Autodesk Inventor part; units mm, degrees
ref_plane "YZ Plane" through (0, 0, 0) normal (1, 0, 0) x (0, 1, 0)
ref_plane "XZ Plane" through (0, 0, 0) normal (0, 1, 0) x (-1, 0, 0)
ref_plane "XY Plane" through (0, 0, 0) normal (0, 0, 1) x (1, 0, 0)
sketch "Sketch1" plane through (0, 0, 0) normal (1, 0, 0) x (0, 1, 0)
  point P0 (0, 0)
sketch "Sketch2" plane through (0, 0, 0) normal (1, 0, 0) x (0, 1, 0)
  line L0 (57.15, 57.15) -> (-57.15, 57.15)
  line L1 (-57.15, 57.15) -> (-57.15, -57.15)
  line L2 (-57.15, -57.15) -> (57.15, -57.15)
  line L3 (57.15, -57.15) -> (57.15, 57.15)
  line L4 (57.15, 57.15) -> (-57.15, -57.15) construction
  line L5 (-57.15, 57.15) -> (57.15, -57.15) construction
  point P0 (0, 0)
  dimension "d0" = 114.3
  dimension "d1" = 114.3
extrude "Extrusion1" add sketch "Sketch2" along normal blind 254
sketch "Sketch3" plane through (0, 57.15, 57.15) normal (0, 1, 0) x (1, 0, 0)
  line L0 (3.9878, 110.3122) -> (250.0122, 110.3122)
  line L1 (250.0122, 110.3122) -> (250.0122, 3.9878)
  line L2 (250.0122, 3.9878) -> (3.9878, 3.9878)
  line L3 (3.9878, 3.9878) -> (3.9878, 110.3122)
  line L4 (0, 114.3) -> (254, 114.3)
  line L5 (0, 114.3) -> (0, 0)
  line L6 (0, 0) -> (254, 0)
  line L7 (254, 114.3) -> (254, 0)
  point P0 (0, 57.15)
  dimension "d4" = 3.9878
  dimension "d5" = 3.9878
  dimension "d6" = 3.9878
  dimension "d7" = 3.9878
extrude "Extrusion2" cut sketch "Sketch3" against normal blind 110.3122 contours L0 L1 L2 L3
sketch "Sketch5" plane through (0, -57.15, 57.15) normal (0, 0, 1) x (1, 0, 0)
  circle A0 centre (57.15, 50.8) radius 5.0038
  circle A1 centre (196.85, 50.8) radius 5.0038
  line L0 (0, 0) -> (254, 0)
  line L1 (0, 114.3) -> (0, 0)
  line L2 (254, 114.3) -> (254, 0)
  point P0 (0, 57.15)
  dimension "d19" = 10.0076
  dimension "d20" = 10.0076
  dimension "d21" = 50.8
  dimension "d22" = 50.8
  dimension "d23" = 57.15
  dimension "d24" = 57.15
extrude "Extrusion3" cut sketch "Sketch5" against normal through all
sketch "Sketch6" plane through (0, -57.15, -57.15) normal (0, -1, 0) x (1, 0, 0)
  circle A0 centre (50.8, 57.15) radius 1.9939
  circle A1 centre (76.2, 57.15) radius 1.9939
  circle A2 centre (177.8, 57.15) radius 1.9939
  circle A3 centre (203.2, 57.15) radius 1.9939
  line L0 (0, 114.3) -> (254, 114.3)
  line L1 (0, 114.3) -> (0, 0)
  line L2 (254, 114.3) -> (254, 0)
  point P0 (0, 57.15)
  dimension "d27" = 3.9878
  dimension "d28" = 3.9878
  dimension "d29" = 3.9878
  dimension "d30" = 3.9878
  dimension "d31" = 57.15
  dimension "d32" = 57.15
  dimension "d33" = 57.15
  dimension "d34" = 57.15
  dimension "d35" = 50.8
  dimension "d36" = 50.8
  dimension "d37" = 76.2
  dimension "d38" = 76.2
extrude "Extrusion4" cut sketch "Sketch6" against normal through all
fillet "Fillet3" radius 1.999 4 edges at (250.0122, 57.15, 0) (127, 57.15, -53.1622) (127, 57.15, 53.1622) (3.9878, 57.15, 0)
sketch "Sketch7" plane through (0, 0, 0) normal (-1, 0, 0) x (0, 0, 1)
  circle A0 centre (-27.1526, 27.1526) radius 9.9949
  circle A1 centre (27.1526, 27.1526) radius 9.9949
  line L0 (-31.75, -11.7602) -> (31.75, -11.7602)
  line L1 (31.75, -11.7602) -> (31.75, -31.75)
  line L2 (31.75, -31.75) -> (-31.75, -31.75)
  line L3 (-31.75, -31.75) -> (-31.75, -11.7602)
  line L4 (57.15, -57.15) -> (-57.15, -57.15)
  line L5 (57.15, 57.15) -> (57.15, -57.15)
  line L6 (-57.15, 57.15) -> (57.15, 57.15)
  line L7 (-57.15, -57.15) -> (-57.15, 57.15)
  point P0 (0, 0)
  dimension "d43" = 19.9898
  dimension "d44" = 19.9898
  dimension "d45" = 63.5
  dimension "d46" = 19.9898
  dimension "d47" = 25.4
  dimension "d48" = 25.4
  dimension "d49" = 29.9974
  dimension "d50" = 29.9974
  dimension "d51" = 29.9974
  dimension "d52" = 29.9974
sketch "Sketch8" plane through (0, 0, 0) normal (-1, 0, 0) x (0, 0, 1)
  point P0 (0, 0)
extrude "Extrusion5" cut sketch "Sketch7" against normal blind 3.9878 contours A0 | A1 | L0 L1 L2 L3
sketch "Sketch9" plane through (254, 0, 0) normal (1, 0, 0) x (0, 0, -1)
  circle A0 centre (-38.1, 38.1) radius 1.9939
  circle A1 centre (38.1, 38.1) radius 1.9939
  circle A2 centre (-38.1, -38.1) radius 1.9939
  circle A3 centre (38.1, -38.1) radius 1.9939
  line L0 (57.15, 57.15) -> (-57.15, 57.15)
  line L1 (-57.15, 57.15) -> (-57.15, -57.15)
  line L2 (57.15, -57.15) -> (57.15, 57.15)
  line L3 (-57.15, -57.15) -> (57.15, -57.15)
  point P0 (0, 0)
  dimension "d55" = 3.9878
  dimension "d56" = 3.9878
  dimension "d57" = 3.9878
  dimension "d58" = 3.9878
  dimension "d59" = 19.05
  dimension "d60" = 19.05
  dimension "d61" = 19.05
  dimension "d62" = 19.05
  dimension "d63" = 19.05
  dimension "d64" = 19.05
  dimension "d65" = 19.05
  dimension "d66" = 19.05
sketch "Sketch10" plane through (254, 0, 0) normal (1, 0, 0) x (0, 0, -1)
  point P0 (0, 0)
extrude "Extrusion6" cut sketch "Sketch9" against normal blind 3.9878 contours A0 | A1 | A2 | A3
sketch "Sketch16" plane through (0, -57.15, 57.15) normal (0, 0, 1) x (1, 0, 0)
  point P0 (0, 57.15)
sketch "Sketch17" plane through (0, -57.15, 57.15) normal (0, 0, 1) x (1, 0, 0)
  point P0 (0, 57.15)
sketch "Sketch18" plane through (0, 0, 0) normal (-1, 0, 0) x (0, 0, 1)
  circle A0 centre (0, 31.75) radius 1.9939
  circle A1 centre (0, -44.45) radius 1.9939
  line L0 (-57.15, 57.15) -> (57.15, 57.15)
  line L1 (57.15, -57.15) -> (-57.15, -57.15)
  point P0 (0, 0)
  dimension "d89" = 3.9878
  dimension "d90" = 3.9878
  dimension "d91" = 25.4
  dimension "d92" = 12.7
extrude "Extrusion11" add sketch "Sketch18" along normal blind 25.4
sketch "Sketch19" plane through (0, 0, 0) normal (-1, 0, 0) x (0, 0, 1)
  point P0 (0, 0)
properties part number "pranshu part" material "PBT Plastic"
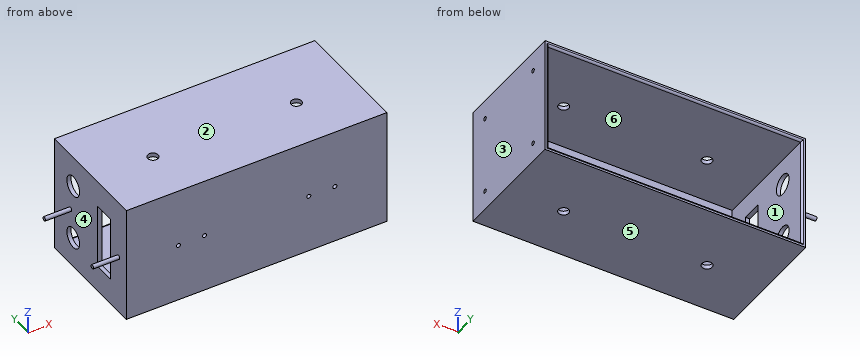
Verification items for the finished model (mm, model axes). Face numbers are marked on the shaded views. A direction names the side the tool comes from. Coordinates: 2 decimals unless noted, no trailing zeros. Write each loop counter-clockwise with the first axis right and the second up, starting at its lowest first coordinate (ties: lowest second). Pieces come first, ordered by that corner, then holes. Notation, with made-up numbers: M 19.25,2 L 49.25,2 A26 ccw 49.25,38 Z; hole C -19.75,41 d7. An arc over 180 degrees is marked long. Use a Markdown table: item, result.
Q1. Sectioned sample at B-B, the plane x = 57.15. Record the boundary of the cut face in (y, z).
Reply:
| item | result |
|---|---|
| outline | M -57.15,-57.15 L -11.35,-57.15 L -11.35,-53.16 L -53.16,-53.16 L -53.16,53.16 L -11.35,53.16 L -11.35,57.15 L -57.15,57.15 Z; M -1.35,-57.15 L 57.15,-57.15 L 57.15,-55.16 A2 ccw 55.15,-53.16 L -1.35,-53.16 Z; M -1.35,53.16 L 55.15,53.16 A2 ccw 57.15,55.16 L 57.15,57.15 L -1.35,57.15 Z |
Q2. Draft check along X on the marked faces 1, 2, 3 and 4. Enter one of: +X half, -X half, draft (parallel to the pull), parting line (faces both ways), or undercut.
Reply:
| item | result |
|---|---|
| face 1 | undercut |
| face 2 | draft |
| face 3 | +X half |
| face 4 | -X half |
Q3. Set-up check for the marked faces 5 and 6: record each of +Z, -Z, +X, -X, +Y, -Y from which the full face is reachable in a straight line by a thin tool's end or side.
Reply:
| item | result |
|---|---|
| face 5 | -Z, +X, -X, +Y, -Y |
| face 6 | +Y |
Q4. Sectioned sample at A-A, the plane y = 3. Record the boundary of the cut face in (x, z), plus the area to 3 significant figures.
Reply:
| item | result |
|---|---|
| outline | M 0,-57.15 L 254,-57.15 L 254,57.15 L 0,57.15 Z; hole M 3.99,-53.16 L 250.01,-53.16 L 250.01,53.16 L 3.99,53.16 Z |
| area | 2,870 mm² |
Q5. Sectioned sample at C-C, the plane z = -46.5. Record the boundary of the cut face in (x, y), plus the area to 3 significant figures.
Reply:
| item | result |
|---|---|
| outline | M 0,-57.15 L 254,-57.15 L 254,57.15 L 252.01,57.15 A2 ccw 250.01,55.15 L 250.01,-53.16 L 3.99,-53.16 L 3.99,55.15 A2 ccw 1.99,57.15 L 0,57.15 Z |
| area | 1,890 mm² |
Q6. Go/stop test with flat-tipped pins: P1, Ø1, axis at x = 209.5, z = -36.5, coming from the +Y side; P2, Ø10, axis at y = 22.5, z = 25, coming from the -X side; P3, Ø2.5, axis at y = 38.1, z = -38.1, coming from the +X side. Record where each tip stops, or that it passes through.
Reply:
| item | result |
|---|---|
| P1 | stops at y = -53.16 |
| P2 | stops at x = 0 |
| P3 | stops at x = 3.99 |
Q7. Thickness scan on line 1 (X direction, y = -6, z = 55); line 2 (X direction, y = -33.5, z = -27); line 3 (Z direction, x = 138, y = -8.5). Record the ranges inside material, lowest first.
Reply:
| item | result |
|---|---|
| line 1 | x = 0 to 52.16, 62.14 to 191.86, 201.84 to 254 |
| line 2 | x = 0 to 3.99, 250.01 to 254 |
| line 3 | z = -57.15 to -53.16, 53.16 to 57.15 |
Q8. Sectioned sample at D-D, the plane x = 136. Record the boundary of the cut face in (y, z).
Reply:
| item | result |
|---|---|
| outline | M -57.15,-57.15 L 57.15,-57.15 L 57.15,-55.16 A2 ccw 55.15,-53.16 L -53.16,-53.16 L -53.16,53.16 L 55.15,53.16 A2 ccw 57.15,55.16 L 57.15,57.15 L -57.15,57.15 Z |
